from build123d import *

# Parameters (mm, degrees)
ESQUISSE1_R                  = 300
BOSS_EXTRU_1_DEPTH           = 22
ESQUISSE2_R                  = 4
ENL_V_MAT_EXTRU_1_DEPTH      = 23
R_P_TITION_CIRCULAIRE1_COUNT = 4
ESQUISSE4_R                  = 12
ENL_V_MAT_EXTRU_2_DEPTH      = 5


with BuildPart() as part:
    # Esquisse1 → Boss.-Extru.1 (new body)
    with BuildSketch(Plane.XY):
        Circle(ESQUISSE1_R)
    extrude(amount=BOSS_EXTRU_1_DEPTH)

    # Esquisse2 → Enlèv. mat.-Extru.1 (cut, through all)
    with BuildSketch(Plane.XY.offset(22)):
        with Locations((0, 280)):
            Circle(ESQUISSE2_R)
    enl_v_mat_extru_1 = extrude(amount=-ENL_V_MAT_EXTRU_1_DEPTH, mode=Mode.SUBTRACT)

    # Répétition circulaire1: Enlèv. mat.-Extru.1 ×4 about axis
    r_p_tition_circulaire1_axis = Axis((0, 0, 0), (0, 0, 1))
    for i in range(1, R_P_TITION_CIRCULAIRE1_COUNT):
        add(enl_v_mat_extru_1.rotate(r_p_tition_circulaire1_axis, i * 360 / R_P_TITION_CIRCULAIRE1_COUNT), mode=Mode.SUBTRACT)

    # Esquisse4 → Enlèv. mat.-Extru.2 (cut)
    with BuildSketch(Plane(origin=(0, 0, 0), x_dir=(-1, 0, 0), z_dir=(0, 0, -1))):
        with Locations((0, 280)):
            Circle(ESQUISSE4_R)
    extrude(amount=-ENL_V_MAT_EXTRU_2_DEPTH, mode=Mode.SUBTRACT)


solid = part.part
Input: part model. Units: mm. Frame: model coordinates. A direction names the side the tool comes from. Coordinates: 2 decimals unless noted, no trailing zeros. Loops run counter-clockwise (first coordinate to the right, second up) from the corner with the lowest first, then second, coordinate; pieces in that order, holes last.
Q1. Material intervals for line 1 (Y direction, x = 0, z = 11.25); line 2 (X direction, y = -0.5, z = 13.5); line 3 (Y direction, x = 188, z = 17.75), sorted ascending.
Q2. Draft query along Y for faces 1 (the face through (-4, 4, 22)), 2 (the face through (2.601, 268.285, 2.465)), 3 (the face through (-39.054, 297.447, 10.846)). Return one class per face: +Y half, -Y half, draft (parallel to the pull), parting line (faces both ways), or undercut.
Q3. Cut plane C-C (x = -262). Output: boundary loops of the cut face in (y, z), then the cut area to 3 significant figures.
Q4. Cut plane A-A (z = 12.25). Output: boundary loops of the cut face in (x, y), then the cut area to 3 significant figures.
Q5. Set-up query: faces 4 (the face through (-4, 4, 0)), 5 (the face through (3, 283, 5)). Return all of +Z, -Z, +X, -X, +Y, -Y with unobstructed straight access to the full face (end or side cutting, diameter ignored); none if empty.
Q6. Contact query for flat-ended pins moving along their axis: pin 1 (3 mm diameter, centred on y = 179.5, z = 17, fed in from +X); pin 2 (6.5 mm diameter, centred on x = 280, y = 0, fed in from +Z); pin 3 (4 mm diameter, centred on y = -93, z = 18, fed in from +X); pin 4 (1 mm diameter, centred on x = -59, z = 14.5, fed in from -Y). Output: stop coordinate, or through.
Q7. Cut plane B-B (y = 170). Output: boundary loops of the cut face in (x, z), then the cut area to 3 significant figures.
Working result:
1. line 1: y = -300 to -284, -276 to 276, 284 to 300
1. line 2: x = -300 to -283.97, -276.03 to 276.03, 283.97 to 300
1. line 3: y = -233.79 to 233.79
2. face 1: draft
2. face 2: undercut
2. face 3: parting line
3. outline: (-146.14, 0) - (146.14, 0) - (146.14, 22) - (-146.14, 22) - close
3. area: 6,430 mm2
4. outline: circle Ø600 at (0, 0); hole circle Ø8 at (-280, 0); hole circle Ø8 at (0, -280); hole circle Ø8 at (0, 280); hole circle Ø8 at (280, 0)
4. area: 283,000 mm2
5. face 4: -Z, +X, -X, +Y, -Y
5. face 5: -Z
6. pin 1: stops at x = 241.49
6. pin 2: passes through
6. pin 3: stops at x = 285.87
6. pin 4: stops at y = -294.24
7. outline: (-247.18, 0) - (247.18, 0) - (247.18, 22) - (-247.18, 22) - close
7. area: 10,900 mm2
